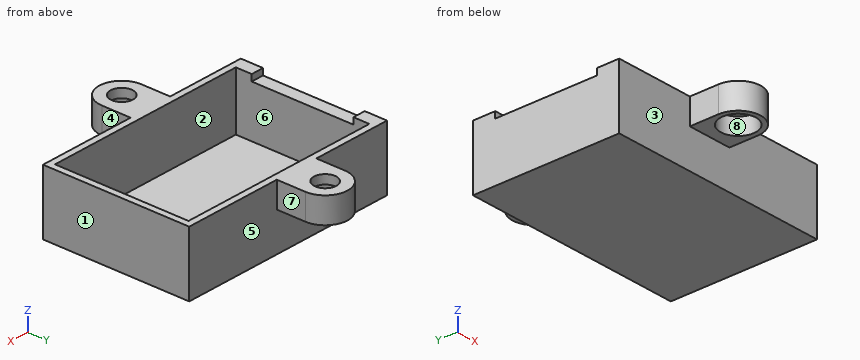
from build123d import *

# Parameters (mm, degrees)
SKETCH270_W         = 32
SKETCH270_H         = 21
PAD127_DEPTH        = 4
SKETCH271_W         = 35
SKETCH271_H         = 23
SKETCH271_W_2       = 32
SKETCH271_H_2       = 21
PAD128_DEPTH        = 10
SKETCH272_W         = 35
SKETCH272_H         = 23
PAD129_DEPTH        = 1
SKETCH273_W         = 16
SKETCH273_H         = 1
POCKET111_DEPTH     = 5
HOLE011_D           = 3.5
HOLE011_DEPTH       = 25
HOLE011_CBORE_D     = 5.5
HOLE011_CBORE_DEPTH = 2.6


with BuildPart() as part:
    # Sketch270 → Pad127 (new body)
    with BuildSketch(Plane(origin=(0, 0, -20), x_dir=(1, 0, 0), z_dir=(0, 0, -1))):
        with BuildLine():
            ThreePointArc((-18.5, 16), (-22, 19.5), (-25.5, 16))
            Line((-25.5, 11.5), (-25.5, 16))
            Line((-25.5, 11.5), (-38, 11.5))
            Line((-38, 11.5), (-38, -11.5))
            Line((-38, -11.5), (-25.5, -11.5))
            Line((-25.5, -11.5), (-25.5, -16))
            ThreePointArc((-25.5, -16), (-22, -19.5), (-18.5, -16))
            Line((-18.5, -11.5), (-18.5, -16))
            Line((-18.5, -11.5), (-3, -11.5))
            Line((-3, 11.5), (-3, -11.5))
            Line((-3, 11.5), (-18.5, 11.5))
            Line((-18.5, 11.5), (-18.5, 16))
        make_face()
        with Locations((-20, 0)):
            Rectangle(SKETCH270_W, SKETCH270_H, mode=Mode.SUBTRACT)
    extrude(amount=PAD127_DEPTH)

    # Sketch271 → Pad128 (join)
    with BuildSketch(Plane(origin=(0, 0, -20), x_dir=(1, 0, 0), z_dir=(0, 0, -1))):
        with Locations((-20.5, 0)):
            Rectangle(SKETCH271_W, SKETCH271_H)
        with Locations((-20, 0)):
            Rectangle(SKETCH271_W_2, SKETCH271_H_2, mode=Mode.SUBTRACT)
    extrude(amount=PAD128_DEPTH)

    # Sketch272 (on Face20 of Pad128) → Pad129 (join)
    with BuildSketch(Plane(origin=(0, 0, -30), x_dir=(1, 0, 0), z_dir=(0, 0, -1))):
        with Locations((-20.5, 0)):
            Rectangle(SKETCH272_W, SKETCH272_H)
    extrude(amount=-PAD129_DEPTH)

    # Sketch273 (on Face12 of Pad129) → Pocket111 (cut)
    with BuildSketch(Plane(origin=(-38, 0, -20), x_dir=(0, 1, 0), z_dir=(-1, 0, 0))):
        with Locations((0, 0.5)):
            Rectangle(SKETCH273_W, SKETCH273_H)
    extrude(amount=-POCKET111_DEPTH, mode=Mode.SUBTRACT)

    # Hole011
    with Locations(Plane(origin=(0, 0, -24), x_dir=(1, 0, 0), z_dir=(0, 0, -1))):
        with Locations((-22, 16), (-22, -16)):
            CounterBoreHole(HOLE011_D / 2, HOLE011_CBORE_D / 2, HOLE011_CBORE_DEPTH, depth=HOLE011_DEPTH)


with BuildPart() as part_1:
    # Body029 placement: moved
    add(part.part.moved(Location((-209, 0, -23))))


solid = part_1.part
The model under review builds one solid part; all positions refer to its coordinate system, in mm. Face numbers are marked on the shaded views. A direction names the side the tool comes from. Round coordinates to 2 decimals unless told otherwise and drop trailing zeros. Order: outer loops, then holes, each group sorted by start corner. A loop starts at its lowest first (then second) coordinate and runs counter-clockwise, first axis right, second up. Notation, with made-up numbers: (-17.5, 46) -> (30.5, 46) arc R24 cw to (30.5, 79) -> close; hole circle Ø5 at (27.25, 20.5). An arc over 180 degrees is marked (long way). Use CSV: the item, a comma, the result in double quotes. Start each with the question number.
(1) Consider section D-D on x = -226. Write out the cut boundary in (y, z), and give its area (3 significant figures).
(2) Insertion check: pin 1 (1.5 mm diameter, centred on x = -230, z = -49, fed in from -Y); pin 2 (6 mm diameter, centred on x = -231.5, y = -15, fed in from -Z); pin 3 (2 mm diameter, centred on y = 15, z = -46.5, fed in from -X). Each pin has a flat end and moves straight along its axis. Give the tip position at first contact, or say it passes through.
(3) Tool access review of the marked faces 4, 5, 6, 7 and 8: name each direction out of +Z, -Z, +X, -X, +Y, -Y from which nothing blocks a thin tool from reaching the whole face with its end or side.
(4) Consider section C-C on y = -17. Write out the cut boundary in (x, z), and give its area (3 significant figures).
(5) Wall thickness on probe 1 along Y at (x, z) = (-231, -45.4); probe 2 along X at (y, z) = (16, -46.15); probe 3 along Y at (x, z) = (-231, -43.7): over which ranges is each line inside the solid? List them lowest first. Write a range as from..to.
(6) Consider section A-A on z = -50.5. Write out the cut boundary in (x, y), and give its area (3 significant figures).
(7) Mouldability with a two-part tool opening along X and no side actions: class the marked faces 1, 2 and 3 as pulls with the +X half, pulls with the -X half, needs draft (parallel to the pull), parting line crosses it, or undercut.
(8) Consider section B-B on x = -231. Write out the cut boundary in (y, z), and give its area (3 significant figures).
Responses:
1,outline,"(-11.5, -53) -> (11.5, -53) -> (11.5, -43) -> (10.5, -43) -> (10.5, -52) -> (-10.5, -52) -> (-10.5, -43) -> (-11.5, -43) -> close"
1,area,"41.0 mm²"
2,pin 1,"y = -11.5"
2,pin 2,"z = -47"
2,pin 3,"x = -234.5"
3,face 4,"+Z, -Z, +X, -Y"
3,face 5,"-Z, +Y"
3,face 6,"+Z"
3,face 7,"+Z, -Z, +X, +Y"
3,face 8,"-Z"
4,outline,"(-234.35, -47) -> (-233.56, -47) -> (-233.56, -44.4) -> (-232.44, -44.4) -> (-232.44, -43) -> (-234.35, -43) -> close; (-229.56, -44.4) -> (-228.44, -44.4) -> (-228.44, -47) -> (-227.65, -47) -> (-227.65, -43) -> (-229.56, -43) -> close"
4,area,"9.49 mm²"
5,probe 1,"-19.5..-18.75, -13.25..-10.5, 10.5..13.25, 18.75..19.5"
5,probe 2,"-234.5..-233.75, -228.25..-227.5"
5,probe 3,"-19.5..-17.75, -14.25..-10.5, 10.5..14.25, 17.75..19.5"
6,outline,"(-247, -11.5) -> (-212, -11.5) -> (-212, 11.5) -> (-247, 11.5) -> close; hole (-245, -10.5) -> (-213, -10.5) -> (-213, 10.5) -> (-245, 10.5) -> close"
6,area,"133 mm²"
7,face 1,"pulls with the +X half"
7,face 2,"undercut"
7,face 3,"needs draft"
8,outline,"(-19.5, -47) -> (-18.75, -47) -> (-18.75, -44.4) -> (-17.75, -44.4) -> (-17.75, -43) -> (-19.5, -43) -> close; (-14.25, -44.4) -> (-13.25, -44.4) -> (-13.25, -47) -> (-11.5, -47) -> (-11.5, -53) -> (11.5, -53) -> (11.5, -47) -> (13.25, -47) -> (13.25, -44.4) -> (14.25, -44.4) -> (14.25, -43) -> (10.5, -43) -> (10.5, -52) -> (-10.5, -52) -> (-10.5, -43) -> (-14.25, -43) -> close; (17.75, -44.4) -> (18.75, -44.4) -> (18.75, -47) -> (19.5, -47) -> (19.5, -43) -> (17.75, -43) -> close"
8,area,"66.6 mm²"
